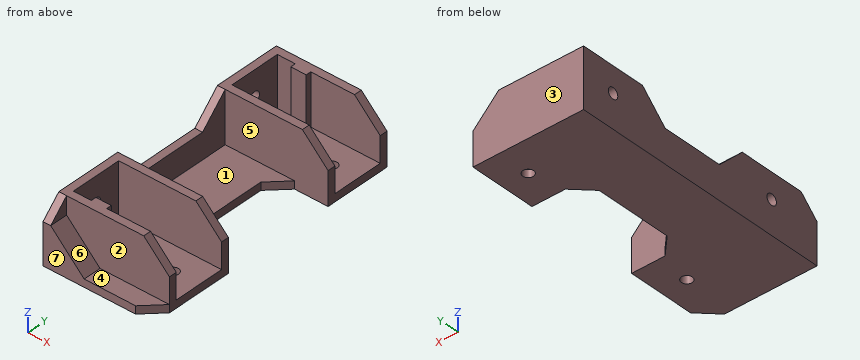
from build123d import *

# Parameters (mm, degrees)
F0_R     = 2.1
F1_DEPTH = 3
F3_DEPTH = 20
F4_R     = 2.1
F5_DEPTH = 3
F7_DEPTH = 7
F9_DEPTH = 103.001


with BuildPart() as f1:
    # F0 (on Top) → F1 (new body)
    with BuildSketch(Plane.XY):
        Polygon((40, 67), (40, 93), (-3, 93), (-3, -10), (33, -10), (40, -3), (40, 23), (27, 23), (20, 30), (20, 60), (27, 67), align=None)
        with Locations((30, 10)):
            Circle(F0_R, mode=Mode.SUBTRACT)
        with Locations((30, 80)):
            Circle(F0_R, mode=Mode.SUBTRACT)
    extrude(amount=F1_DEPTH)

    # F2 (on face) → F3 (join)
    with BuildSketch(Plane.XY.offset(3)):
        Polygon((40, 90), (40, 93), (-3, 93), (-3, -10), (0, -10), (0, -3), (40, -3), (40, 0), (13, 0), (13, 2), (7, 2), (7, 0), (0, 0), (0, 20), (40, 20), (40, 23), (0, 23), (0, 67), (40, 67), (40, 70), (0, 70), (0, 90), (7, 90), (7, 88), (13, 88), (13, 90), align=None)
    extrude(amount=F3_DEPTH)

    # F4 (on face) → F5 (cut, through all)
    with BuildSketch(Plane.YZ):
        with Locations((10, 13)):
            Circle(F4_R)
        Polygon((67, 23), (23, 23), (33, 13), (57, 13), align=None)
        with Locations((80, 13)):
            Circle(F4_R)
        Polygon((-10, 16), (-3, 23), (-10, 23), align=None)
    extrude(amount=-F5_DEPTH, mode=Mode.SUBTRACT)

    # F6 (on face) → F7 (join, through all)
    with BuildSketch(Plane.XZ.offset(10)):
        Polygon((0, 16), (0, 3), (13, 3), align=None)
    extrude(amount=-F7_DEPTH)

    # F8 (on face) → F9 (cut, through all)
    with BuildSketch(Plane(origin=(0, 93, 0), x_dir=(-1, 0, 0), z_dir=(0, 1, 0))):
        Polygon((-30, 23), (-40, 23), (-40, 13), align=None)
    extrude(amount=-F9_DEPTH, mode=Mode.SUBTRACT)


solid = f1.part
Model file for the job. Use its own axes, mm. Face numbers are marked on the shaded views. A direction names the side the tool comes from. Round coordinates to 2 decimals unless told otherwise and drop trailing zeros. Order: outer loops, then holes, each group sorted by start corner. A loop starts at its lowest first (then second) coordinate and runs counter-clockwise, first axis right, second up. Notation, with made-up numbers: M 31.25,-13 L 81.25,-13 A34 cw 81.25,20 Z; hole C -15,27.5 d1. An arc over 180 degrees is marked long. Write each question's results on one line, items separated by ' | '. Start each with the question number.
(1) Saw through at B-B, the plane y = 80. Give the cut face in (x, z).
(2) Saw through at A-A, the plane x = 26. Give the cut face in (y, z), then the cut area to 3 significant figures.
(3) Which spindle directions (+Z, -Z, +X, -X, +Y, -Y) get a long thin tool onto all of the face, cutting with end or side? Do the marked faces 5, 6 and 7. Say none if no direction does.
(4) Two-plate mould, pull along Y, no slides. Class the marked faces 1, 2, 3 and 4: pulls with the +Y half, pulls with the -Y half, needs draft (parallel to the pull), parting line crosses it, or undercut.
(5) Probe probe 1 along Y at (x, z) = (12, 11.75); probe 2 along Y at (x, z) = (32, 17.25); probe 3 along Z at (x, y) = (-0.85, 10). List the from-to ranges inside material, lowest first. Write a range as from..to.
(6) Drop flat-ended pins along their axis: pin 1 (3 mm diameter, centred on x = 16.5, z = 8, fed in from -Y); pin 2 (0.9 mm diameter, centred on y = 45, z = 1, fed in from +X); pin 3 (6 mm diameter, centred on y = 77.5, z = 12.5, fed in from +X). Give the stop position or say it passes through.
(7) Saw through at D-D, the plane x = 12. Give the cut face in (y, z), then the cut area to 3 significant figures.
Established:
1) outline: M -3,0 L 27.9,0 L 27.9,3 L 0,3 L 0,10.9 L -3,10.9 Z; M -3,15.1 L 0,15.1 L 0,23 L -3,23 Z; M 32.1,0 L 40,0 L 40,3 L 32.1,3 Z
2) outline: M -10,0 L 24,0 L 24,3 L 23,3 L 23,23 L 20,23 L 20,3 L 0,3 L 0,23 L -3,23 L -3,3 L -10,3 Z; M 66,0 L 93,0 L 93,23 L 90,23 L 90,3 L 70,3 L 70,23 L 67,23 L 67,3 L 66,3 Z | area: 423 mm^2
3) face 5: +Z, +X | face 6: +Z, +X, -Y | face 7: +Z, -Z, +X, -X, -Y
4) face 1: undercut | face 2: pulls with the -Y half | face 3: pulls with the +Y half | face 4: needs draft
5) probe 1: y = -3..2, 20..23, 67..70, 88..93 | probe 2: y = -3..0, 20..23, 67..70, 90..93 | probe 3: z = 0..10.9, 15.1..23
6) pin 1: stops at y = -3 | pin 2: stops at x = 20 | pin 3: stops at x = 0
7) outline: M -10,0 L 93,0 L 93,23 L 88,23 L 88,3 L 70,3 L 70,23 L 67,23 L 67,3 L 23,3 L 23,23 L 20,23 L 20,3 L 2,3 L 2,23 L -3,23 L -3,4 L -10,4 Z | area: 636 mm^2
